Build history of the part. All positions in model axes, mm. Round coordinates to 2 decimals unless told otherwise and drop trailing zeros. Order: outer loops, then holes, each group sorted by start corner. A loop starts at its lowest first (then second) coordinate and runs counter-clockwise, first axis right, second up. Notation, with made-up numbers: (57, -5) -> (114, -5) arc R16 ccw to (114, 3) -> close; hole circle Ø4 at (67.25, 24.25). An arc over 180 degrees is marked (long way). Use a Markdown table: item, result. Add a question column.
Item 1: Slice it at D-D, the plane z = -50.8. Give the cut face in (x, y) (3 decimals).
Item 2: Probe L1, parallel to X at y = 4.5, z = -50.8 (3 decimals); L2, parallel to Z at x = 122.5, y = 1 (3 decimals); L3, parallel to X at y = 0.5, z = -46.5 (3 decimals). List the from-to ranges inside material, lowest first.
Item 3: Slice it at A-A, the plane z = -87. Give the cut face in (x, y) (3 decimals).
Item 4: Slice it at B-B, the plane x = 25.4. Give the cut face in (y, z).
Item 5: Pin check, flat tips, straight feed: pin 1 (18.5 mm diameter, centred on x = 25.4, z = -50.8, fed in from -Y); pin 2 (12 mm diameter, centred on x = 35, z = -62.5, fed in from -Y). Stop position of each tip, or through.
Item 6: Slice it at C-C, the plane y = 4.25. Give the cut face in (x, z) (3 decimals), plus the area to 3 significant figures.
from build123d import *

# Parameters (mm, degrees)
BOSS_EXTRUDE1_DEPTH = 6.35
SKETCH2_R           = 15.24
CUT_EXTRUDE1_DEPTH  = 294.064711284


with BuildPart() as part:
    # Sketch1 → Boss-Extrude1 (new body)
    with BuildSketch(Plane(origin=(0, 0, 0), x_dir=(1, 0, 0), z_dir=(0, 1, 0))):
        with BuildLine():
            Line((3.81, 0), (250.19, 0))
            ThreePointArc((250.19, 0), (252.884076836, 1.115923164), (254, 3.81))
            Line((254, 3.81), (254, 142.24))
            ThreePointArc((254, 142.24), (252.884076836, 144.934076836), (250.19, 146.05))
            Line((250.19, 146.05), (3.81, 146.05))
            ThreePointArc((3.81, 146.05), (1.115923164, 144.934076836), (0, 142.24))
            Line((0, 142.24), (0, 3.81))
            ThreePointArc((0, 3.81), (1.115923164, 1.115923164), (3.81, 0))
        make_face()
        with BuildLine():
            Line((51.435, 132.715), (202.565, 132.715))
            ThreePointArc((202.565, 132.715), (205.259076836, 131.599076836), (206.375, 128.905))
            Line((206.375, 128.905), (206.375, 17.145))
            ThreePointArc((206.375, 17.145), (205.259076836, 14.450923164), (202.565, 13.335))
            Line((202.565, 13.335), (51.435, 13.335))
            ThreePointArc((51.435, 13.335), (48.740923164, 14.450923164), (47.625, 17.145))
            Line((47.625, 17.145), (47.625, 128.905))
            ThreePointArc((47.625, 128.905), (48.740923164, 131.599076836), (51.435, 132.715))
        make_face(mode=Mode.SUBTRACT)
    extrude(amount=BOSS_EXTRUDE1_DEPTH)

    # Sketch2 → Cut-Extrude1 (cut, through all)
    with BuildSketch(Plane(origin=(0, 6.35, 0), x_dir=(1, 0, 0), z_dir=(0, 1, 0))):
        with Locations(Location((25.4, 50.8, 0), (0, 0, 270))):
            Circle(SKETCH2_R)
        with Locations(Location((228.6, 50.8, 0), (0, 0, 270))):
            Circle(SKETCH2_R)
    extrude(amount=-CUT_EXTRUDE1_DEPTH, mode=Mode.SUBTRACT)


solid = part.part
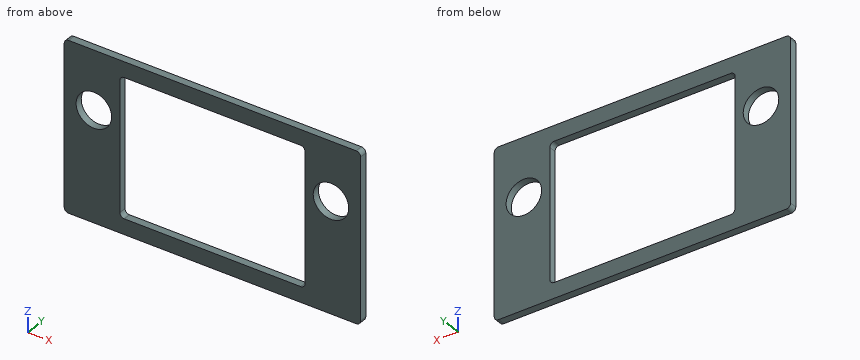
Check sheet entries:
| question | item | result |
|---|---|---|
| 1 | outline | (0, 0) -> (10.16, 0) -> (10.16, 6.35) -> (0, 6.35) -> close; (40.64, 0) -> (47.625, 0) -> (47.625, 6.35) -> (40.64, 6.35) -> close; (206.375, 0) -> (213.36, 0) -> (213.36, 6.35) -> (206.375, 6.35) -> close; (243.84, 0) -> (254, 0) -> (254, 6.35) -> (243.84, 6.35) -> close |
| 2 | L1 | 0 to 10.16, 40.64 to 47.625, 206.375 to 213.36, 243.84 to 254 |
| 2 | L2 | -146.05 to -132.715, -13.335 to 0 |
| 2 | L3 | 0 to 10.779, 40.021 to 47.625, 206.375 to 213.979, 243.221 to 254 |
| 3 | outline | (0, 0) -> (47.625, 0) -> (47.625, 6.35) -> (0, 6.35) -> close; (206.375, 0) -> (254, 0) -> (254, 6.35) -> (206.375, 6.35) -> close |
| 4 | outline | (0, -146.05) -> (6.35, -146.05) -> (6.35, -66.04) -> (0, -66.04) -> close; (0, -35.56) -> (6.35, -35.56) -> (6.35, 0) -> (0, 0) -> close |
| 5 | pin 1 | through |
| 5 | pin 2 | y = 0 |
| 6 | outline | (0, -142.24) arc R3.81 ccw to (3.81, -146.05) -> (250.19, -146.05) arc R3.81 ccw to (254, -142.24) -> (254, -3.81) arc R3.81 ccw to (250.19, 0) -> (3.81, 0) arc R3.81 ccw to (0, -3.81) -> close; hole circle Ø30.48 at (25.4, -50.8); hole (47.625, -128.905) arc R3.81 ccw to (51.435, -132.715) -> (202.565, -132.715) arc R3.81 ccw to (206.375, -128.905) -> (206.375, -17.145) arc R3.81 ccw to (202.565, -13.335) -> (51.435, -13.335) arc R3.81 ccw to (47.625, -17.145) -> close; hole circle Ø30.48 at (228.6, -50.8) |
| 6 | area | 16,700 mm2 |
